Build history of the part. All positions in model axes, mm. A direction names the side the tool comes from. Coordinates: 2 decimals unless noted, no trailing zeros. Loops run counter-clockwise (first coordinate to the right, second up) from the corner with the lowest first, then second, coordinate; pieces in that order, holes last.
Item 1: Cut at B-B (z = 0). List the corners of the cut face in (x, y), and give its area (3 significant figures).
Item 2: Drill centre lines: line 1 along Z through (x, y) = (0, -14.5); line 2 along Y through (x, z) = (1.2, 0.8); line 3 along Z through (x, y) = (-0.7, -8). Where is each one in solid material? Low to high.
Item 3: Mould opens along X. For faces 1 (the face through (0, -20.32, 0)), 2 (the face through (-1.05, -76.2, 0.03)), 3 (the face through (2.286, -38, 0)) say: released by +X, released by -X, zero draft, split by the parting line, or undercut.
Item 4: Cut at C-C (x = 0). List the corners of the cut face in (y, z), and give its area (3 significant figures).
Item 5: Cut at D-D (y = -77). List the corners of the cut face in (x, z), and give its area (3 significant figures).
Item 6: Cut at A-A (y = -10). List the corners of the cut face in (x, z), and give its area (3 significant figures).
Item 7: 3-axis set-ups, long thin cutter, end or side, ignore diameter. For faces 4 (the face through (0, -38, -2.286)), 5 (the face through (0.726, -10.018, -0.556)), 6 (the face through (0.836, -82.461, 0.263)): which of +Z, -Z, +X, -X, +Y, -Y reach the whole face in a straight line?
from build123d import *

# Parameters (mm, degrees)
F0_W     = 4.572
F0_H     = 4.572
F1_DEPTH = 76.2
F2_R     = 0.8763
F3_DEPTH = 12.7
F4_R     = 0.9144
F5_DEPTH = 20.32


with BuildPart() as f1:
    # F0 (on Front) → F1 (new body)
    with BuildSketch(Plane.XZ):
        Rectangle(F0_W, F0_H)
    extrude(amount=F1_DEPTH)

    # F2 (on face) → F3 (join)
    with BuildSketch(Plane.XZ.offset(76.2)):
        Circle(F2_R)
    extrude(amount=F3_DEPTH)

    # F4 (on face) → F5 (cut)
    with BuildSketch(Plane(origin=(0, 0, 0), x_dir=(-1, 0, 0), z_dir=(0, 1, 0))):
        Circle(F4_R)
    extrude(amount=-F5_DEPTH, mode=Mode.SUBTRACT)


solid = f1.part
Filled sheet:
1. outline: (-2.29, -76.2) - (-0.88, -76.2) - (-0.88, -88.9) - (0.88, -88.9) - (0.88, -76.2) - (2.29, -76.2) - (2.29, 0) - (0.91, 0) - (0.91, -20.32) - (-0.91, -20.32) - (-0.91, 0) - (-2.29, 0) - close
1. area: 333 mm2
2. line 1: z = -2.29 to -0.91, 0.91 to 2.29
2. line 2: y = -76.2 to 0
2. line 3: z = -2.29 to -0.59, 0.59 to 2.29
3. face 1: undercut
3. face 2: zero draft
3. face 3: released by +X
4. outline: (-88.9, -0.88) - (-76.2, -0.88) - (-76.2, -2.29) - (0, -2.29) - (0, -0.91) - (-20.32, -0.91) - (-20.32, 0.91) - (0, 0.91) - (0, 2.29) - (-76.2, 2.29) - (-76.2, 0.88) - (-88.9, 0.88) - close
4. area: 333 mm2
5. outline: circle Ø1.75 at (0, 0)
5. area: 2.41 mm2
6. outline: (-2.29, -2.29) - (2.29, -2.29) - (2.29, 2.29) - (-2.29, 2.29) - close; hole circle Ø1.83 at (0, 0)
6. area: 18.3 mm2
7. face 4: -Z, +X, -X, +Y, -Y
7. face 5: +Y
7. face 6: -Y
